```python
from build123d import *

# Parameters (mm, degrees)
SKETCH1_R           = 5
SKETCH1_R_2         = 30
BOSS_EXTRUDE1_DEPTH = 6


with BuildPart() as part:
    # Sketch1 → Boss-Extrude1 (new body)
    with BuildSketch(Plane.XY):
        with BuildLine():
            Line((-99.136639798, -41.760075744), (-58.33663034, 20.302554811))
            ThreePointArc((-58.33663034, 20.302554811), (-52.252875179, 30.168211551), (-46.750843398, 40.36972644))
            Line((-46.750843398, 40.36972644), (-13.40303344, 106.734886383))
            ThreePointArc((-13.40303344, 106.734886383), (0, 115), (13.40303344, 106.734886383))
            Line((13.40303344, 106.734886383), (46.750843398, 40.36972644))
            ThreePointArc((46.750843398, 40.36972644), (52.252875179, 30.168211551), (58.33663034, 20.302554811))
            Line((58.33663034, 20.302554811), (99.136639798, -41.760075744))
            ThreePointArc((99.136639798, -41.760075744), (99.592921435, -57.5), (85.733606358, -64.974810639))
            Line((85.733606358, -64.974810639), (11.585786942, -60.672281251))
            ThreePointArc((11.585786942, -60.672281251), (0, -60.336423102), (-11.585786942, -60.672281251))
            Line((-11.585786942, -60.672281251), (-85.733606358, -64.974810639))
            ThreePointArc((-85.733606358, -64.974810639), (-99.592921435, -57.5), (-99.136639798, -41.760075744))
        make_face()
        with Locations((0, 100)):
            Circle(SKETCH1_R, mode=Mode.SUBTRACT)
        with Locations((86.602540378, -50)):
            Circle(SKETCH1_R, mode=Mode.SUBTRACT)
        with Locations((-86.602540378, -50)):
            Circle(SKETCH1_R, mode=Mode.SUBTRACT)
        Circle(SKETCH1_R_2, mode=Mode.SUBTRACT)
        with Locations((-33.75, 25.061076609)):
            Circle(SKETCH1_R, mode=Mode.SUBTRACT)
        with Locations((33.75, 25.061076609)):
            Circle(SKETCH1_R, mode=Mode.SUBTRACT)
        with Locations((-20, -36.932370625)):
            Circle(SKETCH1_R, mode=Mode.SUBTRACT)
        with Locations((20, -36.932370625)):
            Circle(SKETCH1_R, mode=Mode.SUBTRACT)
    extrude(amount=BOSS_EXTRUDE1_DEPTH)


solid = part.part
```
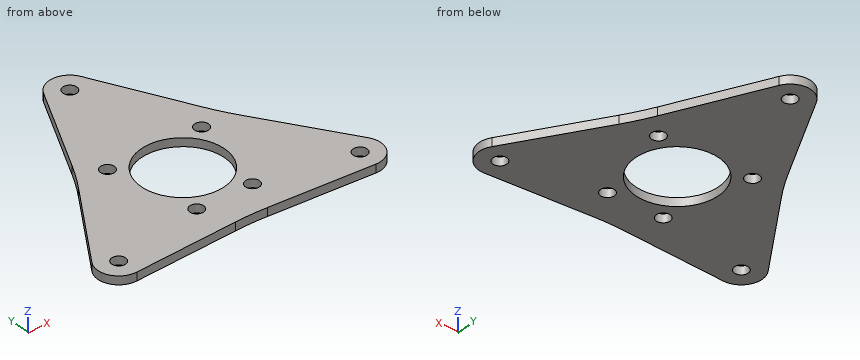
Read the model definition and answer for the solid it produces. Units are mm, in the model's axes. Coordinates: 2 decimals unless noted, no trailing zeros. Order: outer loops, then holes, each group sorted by start corner. A loop starts at its lowest first (then second) coordinate and runs counter-clockwise, first axis right, second up. Notation, with made-up numbers: (-1.75, 10.25) - (51.25, 10.25) arc R18 cw to (51.25, 20.25) - close; hole circle Ø1 at (-4, 0). An arc over 180 degrees is marked (long way). Answer as a JSON object with one key per item and string values. Group by question number.
Item 1: Consider probe 1 along X at (y, z) = (-50.5, 0.45); probe 2 along Y at (x, z) = (84.5, 2.05); probe 3 along X at (y, z) = (97, 3.35). Determine where each line is inside the solid, lowest interval first. Write a range as from..to.
Item 2: Flat-ended cylindrical pins translate along their axes: P1, Ø1, axis at x = 18.5, z = 2, coming from the -Y side; P2, Ø8, axis at x = -33.75, y = 25.06, coming from the -Z side; P3, Ø2, axis at y = 13, z = 2.5, coming from the -X side; P4, Ø1, axis at y = 15, z = 1, coming from the +X side. Find the tip coordinate at first contact, or state that the pin passes through.
Item 3: Section D-D (x = -33.75) is taken. Give the vertices of the cut face in (y, z).
Item 4: Section C-C (y = 17) is taken. Give the vertices of the cut face in (x, z), plus the area to 3 significant figures.
Item 5: Section A-A (y = -50) is taken. Give the vertices of the cut face in (x, z), plus the area to 3 significant figures.
Item 6: Section B-B (x = 0) is taken. Give the vertices of the cut face in (y, z), plus the area to 3 significant figures.
Results are:
{
 "1": {"probe 1": "x = -101.59..-91.58, -81.63..81.63, 91.58..101.59", "probe 2": "y = -64.9..-54.54, -45.46..-19.5", "probe 3": "x = -18.29..-4, 4..18.29"},
 "2": {"P1": "stops at y = -61.1", "P2": "passes through", "P3": "stops at x = -63.79", "P4": "stops at x = 62.15"},
 "3": {"outline": "(-61.96, 0) - (20.06, 0) - (20.06, 6) - (-61.96, 6) - close; (30.06, 0) - (66.24, 0) - (66.24, 6) - (30.06, 6) - close"},
 "4": {"outline": "(-60.51, 0) - (-24.72, 0) - (-24.72, 6) - (-60.51, 6) - close; (24.72, 0) - (60.51, 0) - (60.51, 6) - (24.72, 6) - close", "area": "429 mm^2"},
 "5": {"outline": "(-101.6, 0) - (-91.6, 0) - (-91.6, 6) - (-101.6, 6) - close; (-81.6, 0) - (81.6, 0) - (81.6, 6) - (-81.6, 6) - close; (91.6, 0) - (101.6, 0) - (101.6, 6) - (91.6, 6) - close", "area": "1,100 mm^2"},
 "6": {"outline": "(-60.34, 0) - (-30, 0) - (-30, 6) - (-60.34, 6) - close; (30, 0) - (95, 0) - (95, 6) - (30, 6) - close; (105, 0) - (115, 0) - (115, 6) - (105, 6) - close", "area": "632 mm^2"}
}
